Check sheet for the modelled part. Datum: model origin and axes. Units: mm. A direction names the side the tool comes from. Coordinates: 2 decimals unless noted, no trailing zeros. Loops run counter-clockwise (first coordinate to the right, second up) from the corner with the lowest first, then second, coordinate; pieces in that order, holes last. Notation, with made-up numbers: M -30,8 L -22,8 A24 cw -22,43 Z; hole C 44,-15 d3. An arc over 180 degrees is marked long. Write each question's results on one line, items separated by ' | '. Start each with the question number.
from build123d import *

# Parameters (mm, degrees)
BOSS_EXTRUDE1_DEPTH = 38.1
SKETCH4_R           = 6.35
CUT_EXTRUDE1_DEPTH  = 83.55
FILLET1_R           = 12.7
FILLET2_R           = 2.54


with BuildPart() as part:
    # Sketch1 → Boss-Extrude1 (new body)
    with BuildSketch(Plane(origin=(0, 0, 0), x_dir=(1, 0, 0), z_dir=(0, 1, 0))):
        Polygon((-11.90625, 27.9796875), (-11.90625, -10.1203125), (70.64375, -10.1203125), (70.64375, 27.9796875), (67.46875, 27.9796875), (67.46875, -6.9453125), (-8.73125, -6.9453125), (-8.73125, 27.9796875), align=None)
    extrude(amount=BOSS_EXTRUDE1_DEPTH)

    # Sketch4 → Cut-Extrude1 (cut, through all)
    with BuildSketch(Plane(origin=(70.64375, 0, 0), x_dir=(0, 0, -1), z_dir=(1, 0, 0))):
        with Locations((8.9296875, 19.05)):
            Circle(SKETCH4_R)
    extrude(amount=-CUT_EXTRUDE1_DEPTH, mode=Mode.SUBTRACT)

    # Fillet1
    fillet1_edges = [part.edges().sort_by_distance(p)[0] for p in [
        (-10.31875, 0, -27.9796875),
        (69.05625, 38.1, -27.9796875),
        (-10.31875, 38.1, -27.9796875),
        (69.05625, 0, -27.9796875),
    ]]
    fillet(fillet1_edges, radius=FILLET1_R)

    # Fillet2
    fillet2_edges = [part.edges().sort_by_distance(p)[0] for p in [
        (-8.73125, 19.05, 6.9453125),
        (67.46875, 19.05, 6.9453125),
        (70.64375, 19.05, 10.1203125),
        (-11.90625, 19.05, 10.1203125),
    ]]
    fillet(fillet2_edges, radius=FILLET2_R)


solid = part.part
1) Section check A-A (y = 19.05). Enter the section's corners in (x, z).
2) Section check C-C (y = 5). Enter the section's corners in (x, z).
3) Section check D-D (x = 47.5). Enter the section's corners in (y, z), then the cut area to 3 significant figures.
4) Thickness scan on probe 1 along X at (y, z) = (31, -14.5); probe 2 along Z at (x, y) = (68, 19); probe 3 along Z at (x, y) = (2, 27.5). Record the ranges inside material, lowest first.
5) Release check for a two-part mould opening along Y. For faces 3 (the flat face through (-8.731, 23, -15)), 4 (the cylindrical face through (69.078, 25.346, -8.103)), 5 (the flat face through (29, 38.1, 9)) record: +Y half, -Y half, draft (parallel to the pull), parting line (faces both ways), or undercut.
6) Section check B-B (z = -11). Enter the section's corners in (x, y), then the cut area to 3 significant figures.
7) Gauge pin test, flat ends, axial feed: P1, Ø4, axis at x = -2, y = 27, coming from the -Z side; P2, Ø11.5, axis at y = 19.05, z = -8.93, coming from the -X side; P3, Ø20.5, axis at y = 19.05, z = -8.93, coming from the -X side. Record the tip position at first contact, or that the pin passes through.
8) Set-up check for faces 1 (the cylindrical face through (66.705, 19.317, 6.221)), 2 (the flat face through (29, 19, 10.12)): record each of +Z, -Z, +X, -X, +Y, -Y from which the full face is reachable in a straight line by a thin tool's end or side.
Return value:
1) outline: M -11.91,-27.98 L -8.73,-27.98 L -8.73,-15.28 L -11.91,-15.28 Z; M -11.91,-2.58 L -8.73,-2.58 L -8.73,4.41 A2.54 cw -6.19,6.95 L 64.93,6.95 A2.54 cw 67.47,4.41 L 67.47,-2.58 L 70.64,-2.58 L 70.64,7.58 A2.54 ccw 68.1,10.12 L -9.37,10.12 A2.54 ccw -11.91,7.58 Z; M 67.47,-27.98 L 70.64,-27.98 L 70.64,-15.28 L 67.47,-15.28 Z
2) outline: M -11.91,-25.38 L -8.73,-25.38 L -8.73,4.41 A2.54 cw -6.19,6.95 L 64.93,6.95 A2.54 cw 67.47,4.41 L 67.47,-25.38 L 70.64,-25.38 L 70.64,7.58 A2.54 ccw 68.1,10.12 L -9.37,10.12 A2.54 ccw -11.91,7.58 Z
3) outline: M 0,6.95 L 38.1,6.95 L 38.1,10.12 L 0,10.12 Z | area: 121 mm2
4) probe 1: x = -11.91 to -8.73, 67.47 to 70.64 | probe 2: z = -27.98 to -15.28, -2.58 to 10.12 | probe 3: z = 6.95 to 10.12
5) face 3: draft | face 4: undercut | face 5: +Y half
6) outline: M -11.91,0 L -8.73,0 L -8.73,13.05 L -11.91,13.05 Z; M -11.91,25.05 L -8.73,25.05 L -8.73,38.1 L -11.91,38.1 Z; M 67.47,0 L 70.64,0 L 70.64,13.05 L 67.47,13.05 Z; M 67.47,25.05 L 70.64,25.05 L 70.64,38.1 L 67.47,38.1 Z | area: 166 mm2
7) P1: stops at z = 6.95 | P2: passes through | P3: stops at x = -11.91
8) face 1: -Z, +Y, -Y | face 2: +Z, +X, -X, +Y, -Y
